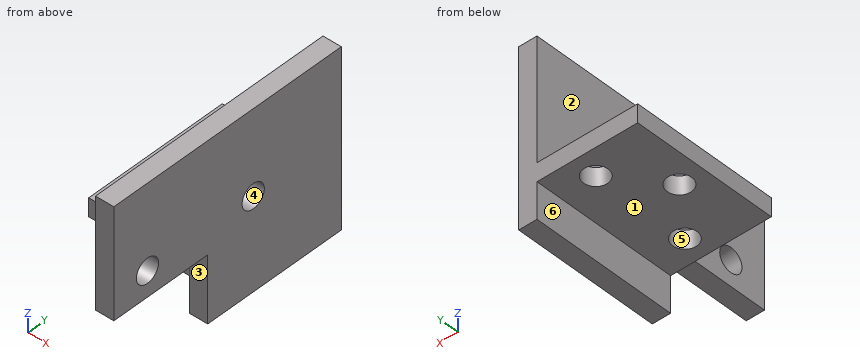
Autodesk Inventor part; units mm, degrees
ref_plane "YZ Plane" through (0, 0, 0) normal (1, 0, 0) x (0, 1, 0)
ref_plane "XZ Plane" through (0, 0, 0) normal (0, 1, 0) x (-1, 0, 0)
ref_plane "XY Plane" through (0, 0, 0) normal (0, 0, 1) x (1, 0, 0)
sketch "Sketch1" plane through (0, 0, 0) normal (0, 0, 1) x (1, 0, 0)
  line L0 (0, 0) -> (16.5, 0)
  line L1 (16.5, 0) -> (16.5, -24)
  line L2 (16.5, -24) -> (0, -24)
  line L3 (0, -24) -> (0, 0)
  line L4 (24.2611, -12.002) -> (-7.0214, -12.002)
  line L5 (10.5138, 0) -> (10.5138, -25.2396)
  line L6 (10.5138, -12.002) -> (10.5138, -20.002) construction
  line L7 (10.5138, -12.002) -> (10.5138, -4.002) construction
  circle A0 centre (10.5138, -4.002) radius 2
  circle A1 centre (10.5138, -20.002) radius 2
  circle A2 centre (4.1138, -12.002) radius 2
  dimension "d0" = 16.5
  dimension "d1" = 24
  dimension "d2" = 8
  dimension "d3" = 8
  dimension "d4" = 4
  dimension "d5" = 4
  dimension "d7" = 4
extrude "Extrusion1" add sketch "Sketch1" along normal blind 3 contours L0 L5 A0 L4 A2 L3 | L0 L1 L4 L5 A0 | L4 A2 L5 A1 L2 L3 | L1 L2 L5 A1 L4
sketch "Sketch2" plane through (16.5, -24, 0) normal (1, 0, 0) x (0, 0, -1)
  line L0 (-3, -16.8669) -> (-3, 24)
  line L1 (-3, -16.8669) -> (-23, -16.8669)
  line L2 (-23, -16.8669) -> (5.9335, -16.8669)
  line L3 (5.9335, -16.8669) -> (5.9335, 24)
  line L4 (5.9335, 24) -> (-23, 24)
  line L5 (-23, 24) -> (-23, -16.8669)
  circle A0 centre (-9.1835, 8.1747) radius 2
  line L6 (-9.1835, 8.1747) -> (-9.1835, -10.8253) construction
  circle A1 centre (-9.1835, -10.8253) radius 2
  dimension "d11" = 20
  dimension "d12" = 4
  dimension "d13" = 19
  dimension "d14" = 4
extrude "Extrusion2" add sketch "Sketch2" along normal blind 3
sketch "Sketch3" plane through (16.5, -24, 0) normal (-1, 0, 0) x (0, 0, 1)
  line L0 (-5.9335, -16.8669) -> (-5.9335, 24)
  line L1 (-5.9335, 0.0047) -> (4.9967, 0.0047)
  line L2 (4.9967, 0.0047) -> (4.9967, -16.8669)
  line L3 (4.9967, -16.8669) -> (-5.9335, -16.8669)
  line L4 (-5.9335, -16.8669) -> (-5.9335, 0.0047)
extrude "Extrusion3" cut sketch "Sketch3" against normal through all
properties part number "bart y endstop v2"
Input: part model. Units: mm. Frame: model coordinates. Face numbers are marked on the shaded views. A direction names the side the tool comes from. Give positions to 0.01 mm unless a question says otherwise; leave off trailing zeros. Order: outer loops, then holes, each group sorted by start corner. A loop starts at its lowest first (then second) coordinate and runs counter-clockwise, first axis right, second up. Notation, with made-up numbers: M -21.5,13 L 33.5,13 A22 ccw 33.5,22 Z; hole C 34,73 d7. An arc over 180 degrees is marked long. Answer as a JSON object with one key per item and string values.
1. Cut plane C-C, the plane z = 8.75. Output: boundary loops of the cut face in (x, y).
Result sheet:
{"outline": "M 16.5,-40.87 L 19.5,-40.87 L 19.5,-36.78 L 16.5,-36.78 Z; M 16.5,-32.87 L 19.5,-32.87 L 19.5,-17.78 L 16.5,-17.78 Z; M 16.5,-13.87 L 19.5,-13.87 L 19.5,0 L 16.5,0 Z"}
2. Ray query, line 1 (Z direction, x = 14.5, y = -22); line 2 (Y direction, x = 17.5, z = 1.25); line 3 (X direction, y = -38, z = 20). Return the intervals inside material, ascending. Write a range as [from, to].
Result sheet:
{"line 1": "[0, 3]", "line 2": "[-24, 0]", "line 3": "[16.5, 19.5]"}
3. Cut plane B-B, the plane y = -34. Output: boundary loops of the cut face in (x, z).
Result sheet:
{"outline": "M 16.5,5 L 19.5,5 L 19.5,7.36 L 16.5,7.36 Z; M 16.5,11.01 L 19.5,11.01 L 19.5,23 L 16.5,23 Z"}
4. Reachability of the marked faces 1, 2 and 3 from +Z, -Z, +X, -X, +Y, -Y: full face, straight path, thin tool, end or side. Return the list, or none.
Result sheet:
{"face 1": "-Z, -X, +Y, -Y", "face 2": "+Z, -X, +Y, -Y", "face 3": "-Z, +X, -X, -Y"}
5. Cut plane A-A, the plane x = 9. Output: boundary loops of the cut face in (y, z), and give its area (3 significant figures).
Result sheet:
{"outline": "M -24,0 L -21.31,0 L -21.31,3 L -24,3 Z; M -18.69,0 L -5.31,0 L -5.31,3 L -18.69,3 Z; M -2.69,0 L 0,0 L 0,3 L -2.69,3 Z", "area": "56.3 mm²"}
6. Cut plane D-D, the plane x = 4.5. Output: boundary loops of the cut face in (y, z), and give its area (3 significant figures).
Result sheet:
{"outline": "M -24,0 L -13.96,0 L -13.96,3 L -24,3 Z; M -10.04,0 L 0,0 L 0,3 L -10.04,3 Z", "area": "60.2 mm²"}
7. Pull-direction query (X, two-part tool) for the marked faces 4, 5 and 6; classes: +X half, -X half, draft (parallel to the pull), parting line (faces both ways), or undercut.
Result sheet:
{"face 4": "draft", "face 5": "undercut", "face 6": "-X half"}
8. First-contact query: P1, Ø6.5, axis at y = -7.5, z = -3.5, coming from the -X side; P2, Ø3.5, axis at x = 11, z = 2, coming from the -Y side; P3, Ø5, axis at x = 10.51, y = -4, coming from the +Z side. Flat tips, straight axial feed; report the tip coordinate or a pass-through.
Result sheet:
{"P1": "x = 16.5", "P2": "y = -24", "P3": "z = 3"}
